Answer from the drawing. Dimensions are ordinates in mm from the lowest x, y and z of the part. Give positions to 0.01 mm unless a question says otherwise; leave off trailing zeros. Write each loop counter-clockwise with the first axis right and the second up, starting at its lowest first coordinate (ties: lowest second). Pieces come first, ordered by that corner, then holes.
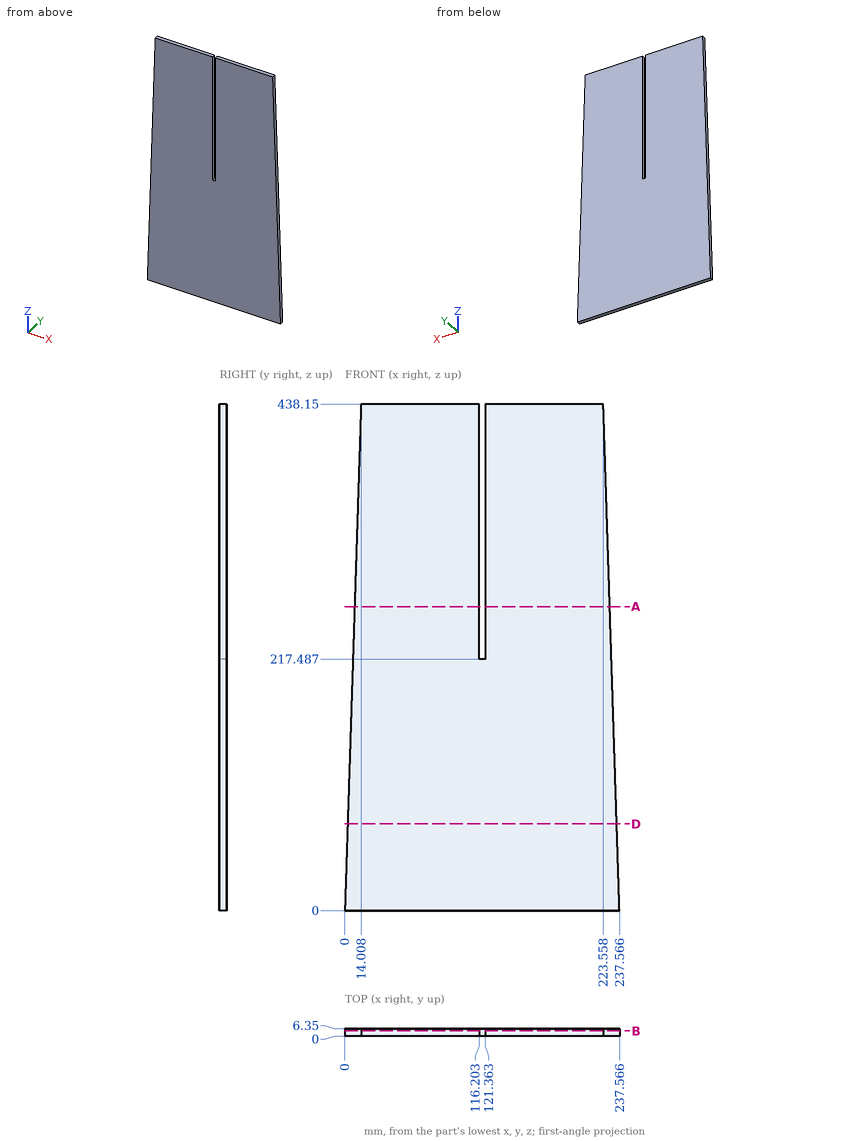
Item 1: Section B-B (y = 4.5) is taken. Write down the section's boundary in (x, z), and give its area (3 significant figures).
Result set:
outline: (0, 0) - (237.57, 0) - (223.56, 438.15) - (121.36, 438.15) - (121.36, 217.49) - (116.2, 217.49) - (116.2, 438.15) - (14.01, 438.15) - close
area: 96,800 mm2
Item 2: Find the intervals of material crossed by line 1 along X through (y, z) = (3.5, 394.5); line 2 along X through (y, z) = (3, 410); line 3 along X through (y, z) = (3.25, 31.5), in increasing order.
Result set:
line 1: x = 12.61 to 116.2, 121.36 to 224.95
line 2: x = 13.11 to 116.2, 121.36 to 224.46
line 3: x = 1.01 to 236.56
Item 3: Section D-D (z = 75) is taken. Write down the section's boundary in (x, y).
Result set:
outline: (2.4, 0) - (235.17, 0) - (235.17, 6.35) - (2.4, 6.35) - close
Item 4: Section A-A (z = 263) is taken. Write down the section's boundary in (x, y), and give its area (3 significant figures).
Result set:
outline: (8.41, 0) - (116.2, 0) - (116.2, 6.35) - (8.41, 6.35) - close; (121.36, 0) - (229.16, 0) - (229.16, 6.35) - (121.36, 6.35) - close
area: 1,370 mm2
Item 5: Each of these flat-tipped pins is pushed along its axis until it touches: pin 1 Ø2 at (y, z) = (4, 329.5) entering from +X; pin 2 Ø1.5 at (y, z) = (3.5, 304) entering from -X (1 decimal); pin 3 Ø3 at (y, z) = (5.5, 207.5) entering from -X. Where does it stop, or does it pass through?
Result set:
pin 1: stops at x = 227.06
pin 2: stops at x = 9.7
pin 3: stops at x = 6.59
